For this review, use the dimensioned drawing (mm, ordinates from the lowest corner) and the shaded views. Coordinates: 2 decimals unless noted, no trailing zeros. Order: outer loops, then holes, each group sorted by start corner. A loop starts at its lowest first (then second) coordinate and runs counter-clockwise, first axis right, second up. Notation, with made-up numbers: M -34.75,5 L -19.75,5 A27 ccw -19.75,36 Z; hole C 46.5,5.25 d11. An arc over 180 degrees is marked long. Answer in a Markdown table with one row per item.
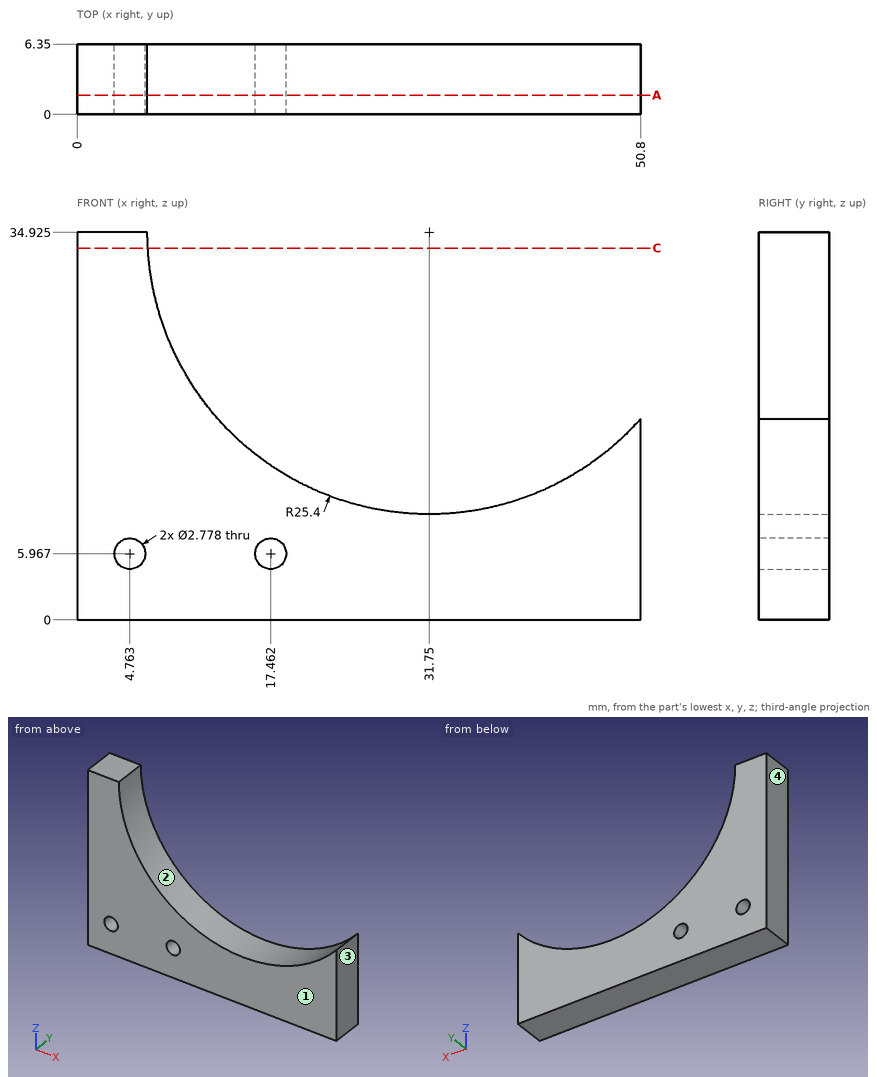
(1) To check wall thickness, follow line 1 (X direction, y = 1.75, z = 7) (1 decimal); line 2 (X direction, y = 2, z = 17) (1 decimal); line 3 (Z direction, x = 30, y = 1) (1 decimal). State the ranges of each line that lie inside material, in increasing order. Write a range as [from, to].
Report:
| item | result |
|---|---|
| line 1 | [0, 3.8], [5.7, 16.5], [18.4, 50.8] |
| line 2 | [0, 13.8], [49.7, 50.8] |
| line 3 | [0, 9.6] |
(2) Take a section at C-C (z = 33.5). Write out the cut boundary in (x, y).
Report:
| item | result |
|---|---|
| outline | M 0,0 L 6.39,0 L 6.39,6.35 L 0,6.35 Z |
(3) Take a section at A-A (y = 1.75). State how many separate pieces and enclosed holes the cut face has, then the cut area to 3 significant figures.
Report:
| item | result |
|---|---|
| separate pieces | 1 |
| enclosed holes | 2 |
| area | 822 mm^2 |
(4) Insertion check: P1, Ø2, axis at x = 34.5, y = 3.5, coming from the -Z side. The pin has a flat end and moves straight along its axis. Give the tip position at first contact, or say it passes through.
Report:
| item | result |
|---|---|
| P1 | z = 0 |
(5) The part is to be moulded in two halves that separate along X. For the marked faces 1, 2, 3 and 4, say which applies: +X half, -X half, draft (parallel to the pull), parting line (faces both ways), or undercut.
Report:
| item | result |
|---|---|
| face 1 | draft |
| face 2 | undercut |
| face 3 | +X half |
| face 4 | -X half |
